Geometry: final body of the model. Coordinates: model frame, mm. A direction names the side the tool comes from. Coordinates: 2 decimals unless noted, no trailing zeros. Order: outer loops, then holes, each group sorted by start corner. A loop starts at its lowest first (then second) coordinate and runs counter-clockwise, first axis right, second up. Notation, with made-up numbers: (60, -3.75) -> (91, -3.75) arc R10 ccw to (91, 3.25) -> close; hole circle Ø11 at (24.25, -36.75). An arc over 180 degrees is marked (long way). Use CSV: the item, a comma, the result in double quotes. Start each with the question number.
Autodesk Inventor part; units mm, degrees
ref_plane "YZ Plane" through (0, 0, 0) normal (1, 0, 0) x (0, 1, 0)
ref_plane "XZ Plane" through (0, 0, 0) normal (0, 1, 0) x (-1, 0, 0)
ref_plane "XY Plane" through (0, 0, 0) normal (0, 0, 1) x (1, 0, 0)
sketch "Sketch1" plane through (0, 0, 0) normal (0, 1, 0) x (-1, 0, 0)
  line L0 (0, 0) -> (-76.2, 0)
  line L1 (-76.2, 0) -> (-76.2, -20)
  line L2 (-76.2, -20) -> (0, -20)
  line L3 (0, -20) -> (0, 0)
  line L4 (0, 0) -> (-76.2, 0)
  line L5 (-76.2, 0) -> (-76.2, -10)
  line L6 (-76.2, -10) -> (0, -10) construction
  line L7 (0, -10) -> (0, 0)
  line L8 (0, -10) -> (-15, -10)
  line L9 (-76.2, -10) -> (-61.2, -10)
  line L10 (-38.1, -10) -> (-38.1, -15)
  dimension "d0" = 20
  dimension "d1" = 76.2
  dimension "d2" = 10
  dimension "d3" = 15
  dimension "d4" = 15
  dimension "d5" = 5
extrude "Extrusion1" add sketch "Sketch1" along normal blind 2
hole "Hole1" at (15, 0, -10) at (38.1, 0, -15) at (61.2, 0, -10) direction (0, 1, 0) diameter 4 depth 10 tip angle 118
sketch "Sketch2" plane through (76.2, 0, 0) normal (1, 0, 0) x (0, 0, -1)
  line L0 (0, 0) -> (0, 1)
  circle A0 centre (0, 1) radius 2
  circle A1 centre (0, 1) radius 1
  dimension "d15" = 1
  dimension "d16" = 4
  dimension "d19" = 2
extrude "Extrusion2" add sketch "Sketch2" against normal blind 76.2
extrude "Extrusion4" cut sketch "Sketch2" against normal blind 76.2 contours A1
properties part number "hinge"
(1) Mould query, pull axis X, two halves, no side actions, for faces 4 (the face through (40.052, 1.014, -14.566)), 5 (the face through (76.2, 1, -9)), 6 (the face through (0, 1, -9)). Classes: pulls with the +X half, pulls with the -X half, needs draft (parallel to the pull), parting line crosses it, or undercut.
(2) First-contact query: pin 1 (10 mm diameter, centred on x = 39.5, z = -8.5, fed in from -Y); pin 2 (10 mm diameter, centred on x = 52.5, z = -10, fed in from +Y); pin 3 (1.5 mm diameter, centred on x = 11, y = 0, fed in from +Z); pin 4 (1.6 mm diameter, centred on y = 1, z = 0, fed in from +X). Flat tips, straight axial feed; report the tip coordinate or a pass-through.
(3) Access query for faces 1 (the face through (39, 0, -11)), 2 (the face through (39, 2, -11)), 3 (the face through (39, 1, -20)). Directions: +Z, -Z, +X, -X, +Y, -Y. A direction counts if a zero-diameter tool reaches every point of the face in a straight line with its end or side. Return the directions, or none.
(4) Line query: line 1 (X direction, y = 0.7, z = -10); line 2 (Z direction, x = 15, y = 1.15); line 3 (Z direction, x = 15, y = 1.4). Output: solid intervals per line, ascending. Write a range as from..to.
(5) Section B-B (y = 1). Return loops of the section in (x, z), then the cut area to 3 significant figures.
(6) Section D-D (z = -8.75). Return loops of the section in (x, y), then the cut area to 3 significant figures.
(7) Section A-A (x = 15). Return loops of the section in (y, z).
(8) Section C-C (z = -0.25). Return loops of the section in (x, y), then the cut area to 3 significant figures.
Check sheet entries:
1,face 4,"undercut"
1,face 5,"pulls with the +X half"
1,face 6,"pulls with the -X half"
2,pin 1,"stops at y = 0"
2,pin 2,"stops at y = 2"
2,pin 3,"stops at z = 1.98"
2,pin 4,"passes through"
3,face 1,"-Z, +X, -X, -Y"
3,face 2,"-Z, +X, -X, +Y"
3,face 3,"-Z, +X, -X, +Y, -Y"
4,line 1,"x = 0..13, 17..59.2, 63.2..76.2"
4,line 2,"z = -20..-12, -8..-0.99, 0.99..1.99"
4,line 3,"z = -20..-12, -8..-0.92, 0.92..1.96"
5,outline,"(0, -20) -> (76.2, -20) -> (76.2, -1) -> (0, -1) -> close; (0, 1) -> (76.2, 1) -> (76.2, 2) -> (0, 2) -> close; hole circle Ø4 at (15, -10); hole circle Ø4 at (38.1, -15); hole circle Ø4 at (61.2, -10)"
5,area,"1,490 mm^2"
6,outline,"(0, 0) -> (13.44, 0) -> (13.44, 2) -> (0, 2) -> close; (16.56, 0) -> (59.64, 0) -> (59.64, 2) -> (16.56, 2) -> close; (62.76, 0) -> (76.2, 0) -> (76.2, 2) -> (62.76, 2) -> close"
6,area,"140 mm^2"
7,outline,"(0, -20) -> (2, -20) -> (2, -12) -> (0, -12) -> close; (0, -8) -> (2, -8) -> (2, -1.73) arc R2 ccw (long way) to (0, -1.73) -> close; hole circle Ø2 at (1, 0)"
8,outline,"(0, -0.98) -> (76.2, -0.98) -> (76.2, 0.03) -> (0, 0.03) -> close; (0, 1.97) -> (76.2, 1.97) -> (76.2, 2.98) -> (0, 2.98) -> close"
8,area,"155 mm^2"
